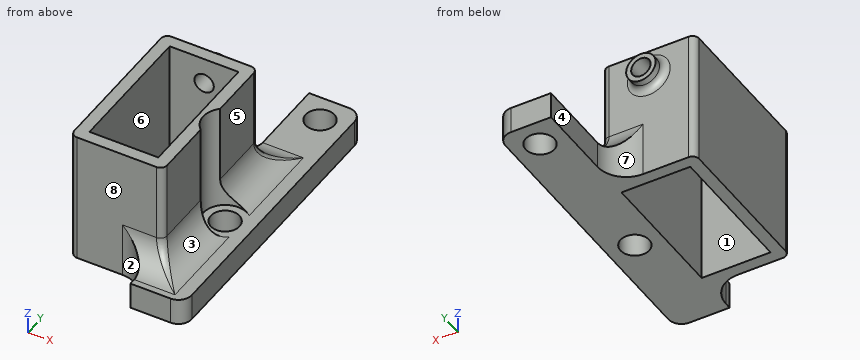
Autodesk Inventor part; units mm, degrees
ref_plane "YZ Plane" through (0, 0, 0) normal (1, 0, 0) x (0, 1, 0)
ref_plane "XZ Plane" through (0, 0, 0) normal (0, 1, 0) x (-1, 0, 0)
ref_plane "XY Plane" through (0, 0, 0) normal (0, 0, 1) x (1, 0, 0)
sketch "Sketch1" plane through (0, 0, 0) normal (0, 0, 1) x (1, 0, 0)
  line L0 (-22.6, 22.6) -> (-14.6, 22.6)
  line L1 (-14.6, 22.6) -> (-14.6, -22.6)
  line L2 (-14.6, -22.6) -> (-22.6, -22.6)
  line L3 (-22.6, -22.6) -> (-22.6, 22.6)
  line L4 (5.4, -5.4) -> (-38.7938, -5.4) construction
  line L5 (-22.6, -5.4) -> (-27.75, -5.4) construction
  line L6 (-32.9, 4.75) -> (-22.6, 4.75)
  line L7 (-22.6, 4.75) -> (-22.6, -15.55)
  line L8 (-22.6, -15.55) -> (-32.9, -15.55)
  line L9 (-32.9, -15.55) -> (-32.9, 4.75)
  line L10 (-32.9, 4.75) -> (-22.6, -15.55) construction
  line L11 (-22.6, 4.75) -> (-32.9, -15.55) construction
  line L12 (-20.8, 6.55) -> (-34.7, 6.55)
  line L13 (-34.7, 6.55) -> (-34.7, -17.35)
  line L14 (-34.7, -17.35) -> (-20.8, -17.35)
  line L15 (-20.8, -17.35) -> (-20.8, 6.55)
  line L16 (-22.6, 22.6) -> (-22.6, 18.6) construction
  line L17 (-22.6, 18.6) -> (-18.6, 18.6) construction
  line L18 (-18.6, 18.6) -> (-18.6, -5.4) construction
  circle A0 centre (-18.6, -5.4) radius 3.3
  circle A1 centre (-18.6, -5.4) radius 2.15
  point P0 (-22.6, 6.55)
  point P1 (-22.6, -17.35)
  point P2 (-20.8, -2.9403)
  point P3 (-20.8, -7.8597)
  dimension "d0" = 8
  dimension "d1" = 45.2
  dimension "d2" = 5.15
  dimension "d3" = 10.3
  dimension "d4" = 20.3
  dimension "d5" = 1.8
  dimension "d10" = 4
  dimension "d11" = 4
  dimension "d12" = 24
  dimension "d32" = 6.6
  dimension "d35" = 4.3
extrude "Extrusion1" add sketch "Sketch1" along normal blind 20 contours L12 L15 A0 L14 L3 | L3 L6 L9 L8 L14 L13 L12 | L15 A0 picked at (-20.9741, -4.7782)
extrude "Extrusion2" add sketch "Sketch1" along normal blind 4 contours L0 L1 L2 L3 L14 L15 A0 L12 | A0 L15 | A1 picked at (-15.7123, -5.1492)
hole "Hole1" at (-18.6, 18.6, 0) at (-18.6, -5.4, 0) direction (0, 0, 1) diameter 4.3 depth 5 tip angle 118
fillet "Fillet1" radius 4.3 5 edges at (-20.8, -5.4, 4) (-21.7, 6.55, 4) (-21.7, -17.35, 4) (-22.6, 6.55, 2) (-22.6, -17.35, 2)
fillet "Fillet3" radius 1 8 edges at (-34.7, 6.55, 10) (-34.7, -17.35, 10) (-23.85, 6.55, 8.3) (-19.55, 10.85, 4) (-20.8, 6.55, 14.15) (-23.85, -17.35, 8.3) (-19.55, -21.65, 4) (-20.8, -17.35, 14.15)
sketch "Sketch2" plane through (-26.9, 6.55, 8.3) normal (0, 1, 0) x (1, 0, 0)
  line L0 (6.1, -11.7) -> (6.1, 0) construction
  line L1 (-7.8, 8.3) -> (-7.8, -11.7) construction
  line L2 (6.1, -11.7) -> (-7.8, -11.7) construction
  line L3 (-7.8, -11.7) -> (-7.8, -3.7) construction
  line L4 (-7.8, -3.7) -> (6.1, -3.7) construction
  line L5 (6.1, -3.7) -> (6.1, -11.7) construction
  line L6 (-7.8, -11.7) -> (6.1, -3.7) construction
  circle A0 centre (-0.85, -7.7) radius 1.45
  circle A1 centre (-0.85, -7.7) radius 2.2
  point P0 (26.9, 8.3)
  dimension "d23" = 8
  dimension "d24" = 2.9
  dimension "d25" = 0.75
extrude "Extrusion3" add sketch "Sketch2" along normal blind 2
fillet "Fillet4" radius 2 2 edges at (-14.6, 22.6, 2) (-14.6, -22.6, 2)
fillet "Fillet5" radius 1 1 edges at (-29.95, 6.55, 16)
extrude "Extrusion4" cut sketch "Sketch2" against normal blind 2 contours A0
extrude "Extrusion5" cut sketch "Sketch1" along normal blind 20 contours A0 L15 | L15 A0 | A1
extrude "Extrusion6" add sketch "Sketch1" along normal blind 4 contours A0 L15 picked at (-15.7123, -5.1492)
extrude "Extrusion7" add sketch "Sketch1" along normal blind 4 contours L15 A0 picked at (-20.9741, -4.7782)
properties material "ABS Plastic"
Design review of the part built by this model. Coordinates are the model's own, in mm. Face numbers are marked on the shaded views. A direction names the side the tool comes from. Give positions to 0.01 mm unless a question says otherwise; leave off trailing zeros. Order: outer loops, then holes, each group sorted by start corner. A loop starts at its lowest first (then second) coordinate and runs counter-clockwise, first axis right, second up. Notation, with made-up numbers: (27, 70) - (69, 70) arc R7 ccw to (69, 79) - close; hole circle Ø1 at (-34, 25.5). An arc over 180 degrees is marked (long way). Use a Markdown table: item, result. Add a question column.
(1) Add section C-C on z = 16. Give the boundary of the cut face in (x, y).
(2) Mouldability with a two-part tool opening along Y and no side actions: class the marked faces 1, 2 and 3 as +Y half, -Y half, draft (parallel to the pull), parting line (faces both ways), or undercut.
(3) Clearance check with flat-ended pins moving along their axes: P1, Ø2, axis at y = 14.5, z = 1.5, coming from the -X side; P2, Ø1.3, axis at x = -28, z = 17, coming from the +Y side; P3, Ø3, axis at x = -27.5, z = 7, coming from the +Y side. State where each tip first meets the part, or that it passes through.
(4) Add section A-A on y = 3. Give the boundary of the cut face in (x, z), then the cut area to 3 significant figures.
(5) Add section B-B on x = -27.75. Give the boundary of the cut face in (y, z), then the cut area to 3 significant figures.
(6) Machinability: for the marked faces 4, 5, 6, 7 and 8, which of the approach directions +Z, -Z, +X, -X, +Y, -Y give a long, thin tool a straight path to every point of the face, cutting with its end or side? Answer none if there is none.
(7) Add section D-D on y = 18.6. Give the boundary of the cut face in (x, z).
(8) Wall thickness on probe 1 along Y at (x, z) = (-18.6, 1); probe 2 along Y at (x, z) = (-29, 5.5); probe 3 along Y at (x, z) = (-26.25, 15.5): over which ranges is each line inside the solid? List them lowest first. Write a range as [from, to].
Report:
| question | item | result |
|---|---|---|
| 1 | outline | (-34.7, -16.35) arc R1 ccw to (-33.7, -17.35) - (-21.8, -17.35) arc R1 ccw to (-20.8, -16.35) - (-20.8, -7.86) arc R3.3 cw to (-20.8, -2.94) - (-20.8, 5.55) arc R1 ccw to (-21.8, 6.55) - (-24.55, 6.55) arc R1 cw to (-25.55, 7.55) - (-25.55, 8.55) - (-26.3, 8.55) - (-26.3, 4.75) - (-22.6, 4.75) - (-22.6, -15.55) - (-32.9, -15.55) - (-32.9, 4.75) - (-29.2, 4.75) - (-29.2, 8.55) - (-29.95, 8.55) - (-29.95, 7.55) arc R1 cw to (-30.95, 6.55) - (-33.7, 6.55) arc R1 ccw to (-34.7, 5.55) - close |
| 2 | face 1 | undercut |
| 2 | face 2 | -Y half |
| 2 | face 3 | draft |
| 3 | P1 | stops at x = -22.6 |
| 3 | P2 | stops at y = 8.55 |
| 3 | P3 | stops at y = 6.65 |
| 4 | outline | (-34.7, 0) - (-32.9, 0) - (-32.9, 20) - (-34.7, 20) - close; (-22.6, 0) - (-14.6, 0) - (-14.6, 4) - (-16.5, 4) arc R4.3 cw to (-20.8, 8.3) - (-20.8, 20) - (-22.6, 20) - close |
| 4 | area | 101 mm² |
| 5 | outline | (-17.35, 0) - (-15.55, 0) - (-15.55, 20) - (-17.35, 20) - close; (4.75, 0) - (6.55, 0) - (6.55, 12.8) arc R1 cw to (7.55, 13.8) - (8.55, 13.8) - (8.55, 14.55) - (4.75, 14.55) - close; (4.75, 17.45) - (8.55, 17.45) - (8.55, 18.2) - (7.55, 18.2) arc R1 cw to (6.55, 19.2) - (6.55, 20) - (4.75, 20) - close |
| 5 | area | 70.2 mm² |
| 6 | face 4 | +Z, -Z, -X, +Y |
| 6 | face 5 | +Z, +X, +Y, -Y |
| 6 | face 6 | +Z, -Z |
| 6 | face 7 | -Z, -X, +Y |
| 6 | face 8 | +Z, -X, -Y |
| 7 | outline | (-22.6, 0) - (-20.75, 0) - (-20.75, 4) - (-22.6, 4) - close; (-16.45, 0) - (-14.6, 0) - (-14.6, 4) - (-16.45, 4) - close |
| 8 | probe 1 | y = [-22.6, -7.55], [-3.25, 16.45], [20.75, 22.6] |
| 8 | probe 2 | y = [-17.35, -15.55], [4.75, 6.55] |
| 8 | probe 3 | y = [-17.35, -15.55], [4.75, 8.55] |
